Could you check a few things on this model? Use its own coordinates, in mm. A direction names the side the tool comes from. Give positions to 0.01 mm unless a question says otherwise; leave off trailing zeros. Order: outer loops, then holes, each group sorted by start corner. A loop starts at its lowest first (then second) coordinate and runs counter-clockwise, first axis right, second up. Notation, with made-up numbers: M 41,19 L 71,19 A19 ccw 71,27 Z; hole C 64.5,62 d10. An arc over 180 degrees is marked long. Answer in a Markdown table with one row per item. Add a question column.
```python
from build123d import *

# Parameters (mm, degrees)
SKETCH1_W           = 10
SKETCH1_H           = 16
BOSS_EXTRUDE1_DEPTH = 3.7
SKETCH2_W           = 8.2
SKETCH2_H           = 14.3
CUT_EXTRUDE1_DEPTH  = 2.7
SKETCH3_W           = 6.6
SKETCH3_H           = 16
CUT_EXTRUDE2_DEPTH  = 1.9
CUT_EXTRUDE3_REACH  = 5.7
SKETCH4_W           = 6.5
SKETCH4_H           = 10
SKETCH5_W           = 5.5
SKETCH5_H           = 16
BOSS_EXTRUDE2_DEPTH = 3.7
CUT_EXTRUDE4_DEPTH  = 4.7


with BuildPart() as part:
    # Sketch1 → Boss-Extrude1 (new body)
    with BuildSketch(Plane(origin=(0, 0, 0), x_dir=(1, 0, 0), z_dir=(0, 1, 0))):
        Rectangle(SKETCH1_W, SKETCH1_H)
    extrude(amount=BOSS_EXTRUDE1_DEPTH)

    # Sketch2 → Cut-Extrude1 (cut)
    with BuildSketch(Plane.XZ):
        Rectangle(SKETCH2_W, SKETCH2_H)
    extrude(amount=-CUT_EXTRUDE1_DEPTH, mode=Mode.SUBTRACT)

    # Sketch3 → Cut-Extrude2 (cut)
    with BuildSketch(Plane.XZ):
        Rectangle(SKETCH3_W, SKETCH3_H)
    extrude(amount=-CUT_EXTRUDE2_DEPTH, mode=Mode.SUBTRACT)

    # Sketch4 → Cut-Extrude3 (cut, up to next)
    with BuildSketch(Plane(origin=(0, 3.7, 0), x_dir=(1, 0, 0), z_dir=(0, 1, 0)), mode=Mode.PRIVATE) as cut_extrude3_sk1:
        Rectangle(SKETCH4_W, SKETCH4_H)
    cut_extrude3_tool1 = extrude(cut_extrude3_sk1.sketch, amount=-CUT_EXTRUDE3_REACH, mode=Mode.PRIVATE) & part.part
    add(cut_extrude3_tool1.solids().sort_by_distance((0, 3.7, 0))[0], mode=Mode.SUBTRACT)

    # Sketch5 → Boss-Extrude2 (add)
    with BuildSketch(Plane.XZ):
        with Locations((-7.75, 0)):
            Rectangle(SKETCH5_W, SKETCH5_H)
    boss_extrude2 = extrude(amount=-BOSS_EXTRUDE2_DEPTH)

    # Sketch6 → Cut-Extrude4 (cut, through all)
    with BuildSketch(Plane(origin=(0, 3.7, 0), x_dir=(1, 0, 0), z_dir=(0, 1, 0))):
        with BuildLine():
            Line((-6.55, 5.55), (-6.55, -5.55))
            ThreePointArc((-6.55, -5.55), (-7.5, -6.5), (-8.45, -5.55))
            Line((-8.45, -5.55), (-8.45, 5.55))
            ThreePointArc((-8.45, 5.55), (-7.5, 6.5), (-6.55, 5.55))
        make_face()
    cut_extrude4 = extrude(amount=-CUT_EXTRUDE4_DEPTH, mode=Mode.SUBTRACT)

    # Mirror1: Boss-Extrude2, Cut-Extrude4 across plane
    add(boss_extrude2.mirror(Plane(origin=(0, 0, 0), x_dir=(0, 0, 1), z_dir=(1, 0, 0))))
    add(cut_extrude4.mirror(Plane(origin=(0, 0, 0), x_dir=(0, 0, 1), z_dir=(1, 0, 0))), mode=Mode.SUBTRACT)


solid = part.part
```
1. For faces 1 (the flat face through (3.3, 0.9, -7.6)), 2 (the flat face through (-3.7, 2.7, 0.1)), 3 (the flat face through (-8.45, 2, 0)), which set-ups out of +Z, -Z, +X, -X, +Y, -Y let a thin tool reach every point of the face, with its end or its side?
2. Thinking about a two-plate mould opening in X: for faces 4 (the flat face through (10.5, 2, 0)), 5 (the flat face through (0, 3, 5)), 6 (the flat face through (0.1, 2.2, -8)), which applies, pulls with the +X half, pulls with the -X half, needs draft (parallel to the pull), parting line crosses it, or undercut?
3. Will these pins go through, and if not, where does the flat tip stop? P1, Ø0.9, axis at x = -1.5, z = 7.5, coming from the -Y side; P2, Ø1.4, axis at x = 0.5, y = 1.5, coming from the -Z side.
4. If I drill on line 1 along X through (y, z) = (2.65, -4); line 2 along X through (y, z) = (3.45, 4.5); line 3 along Z through (x, y) = (2.25, 2.55), over which ranges is the centre line in solid material (lowest first)? Write a range as [from, to].
5. Suppose I cut it at D-D on x = -0.75. List the corners of the cut face in (y, z) for me, plus the area to 3 significant figures.
6. Suppose I cut it at C-C on y = 2.2. List the corners of the cut face in (x, z) for me.
7. Suppose I cut it at A-A on y = 1. List the corners of the cut face in (x, z) for me.
8. Suppose I cut it at B-B on x = -7.5. List the corners of the cut face in (y, z) for me, plus the area to 3 significant figures.
Findings below:
| question | item | result |
|---|---|---|
| 1 | face 1 | +Z, -Z, -Y |
| 1 | face 2 | -Y |
| 1 | face 3 | +Y, -Y |
| 2 | face 4 | pulls with the +X half |
| 2 | face 5 | undercut |
| 2 | face 6 | needs draft |
| 3 | P1 | y = 1.9 |
| 3 | P2 | z = -8 |
| 4 | line 1 | [-10.5, -8.45], [-6.55, -4.1], [4.1, 6.55], [8.45, 10.5] |
| 4 | line 2 | [-10.5, -8.45], [-6.55, -3.25], [3.25, 6.55], [8.45, 10.5] |
| 4 | line 3 | [-8, -7.15], [7.15, 8] |
| 5 | outline | M 1.9,-8 L 3.7,-8 L 3.7,-5 L 2.7,-5 L 2.7,-7.15 L 1.9,-7.15 Z; M 1.9,7.15 L 2.7,7.15 L 2.7,5 L 3.7,5 L 3.7,8 L 1.9,8 Z |
| 5 | area | 7.36 mm2 |
| 6 | outline | M -10.5,-8 L 10.5,-8 L 10.5,8 L -10.5,8 Z; hole M -8.45,-5.55 A0.95 ccw -6.55,-5.55 L -6.55,5.55 A0.95 ccw -8.45,5.55 Z; hole M -4.1,-7.15 L 4.1,-7.15 L 4.1,7.15 L -4.1,7.15 Z; hole M 6.55,-5.55 A0.95 ccw 8.45,-5.55 L 8.45,5.55 A0.95 ccw 6.55,5.55 Z |
| 7 | outline | M -10.5,-8 L -3.3,-8 L -3.3,-7.15 L -4.1,-7.15 L -4.1,7.15 L -3.3,7.15 L -3.3,8 L -10.5,8 Z; M 3.3,-8 L 10.5,-8 L 10.5,8 L 3.3,8 L 3.3,7.15 L 4.1,7.15 L 4.1,-7.15 L 3.3,-7.15 Z; hole M -8.45,-5.55 A0.95 ccw -6.55,-5.55 L -6.55,5.55 A0.95 ccw -8.45,5.55 Z; hole M 6.55,-5.55 A0.95 ccw 8.45,-5.55 L 8.45,5.55 A0.95 ccw 6.55,5.55 Z |
| 8 | outline | M 0,-8 L 3.7,-8 L 3.7,-6.5 L 0,-6.5 Z; M 0,6.5 L 3.7,6.5 L 3.7,8 L 0,8 Z |
| 8 | area | 11.1 mm2 |
